Geometry check sheet. Reference: the model listing, model coordinates, mm. A direction names the side the tool comes from. Give positions to 0.01 mm unless a question says otherwise; leave off trailing zeros. Loops run counter-clockwise (first coordinate to the right, second up) from the corner with the lowest first, then second, coordinate; pieces in that order, holes last.
```python
from build123d import *

# Parameters (mm, degrees)
SKETCH1_R           = 11.1125
BOSS_EXTRUDE1_DEPTH = 18.415
SKETCH2_R           = 4.7625
BOSS_EXTRUDE2_DEPTH = 8.255
SKETCH3_R           = 3.175
BOSS_EXTRUDE3_DEPTH = 12.7
FILLET1_R           = 0.508
FILLET2_R           = 0.508


with BuildPart() as part:
    # Sketch1 → Boss-Extrude1 (new body)
    with BuildSketch(Plane(origin=(0, 0, 0), x_dir=(1, 0, 0), z_dir=(0, 1, 0))):
        with Locations(Location((0, 0, 0), (0, 0, 270))):
            Circle(SKETCH1_R)
    extrude(amount=BOSS_EXTRUDE1_DEPTH)

    # Sketch2 → Boss-Extrude2 (add)
    with BuildSketch(Plane(origin=(0, 18.415, 0), x_dir=(1, 0, 0), z_dir=(0, 1, 0))):
        with Locations(Location((0, 0, 0), (0, 0, 270))):
            Circle(SKETCH2_R)
    extrude(amount=BOSS_EXTRUDE2_DEPTH)

    # Sketch3 → Boss-Extrude3 (add)
    with BuildSketch(Plane(origin=(0, 26.67, 0), x_dir=(1, 0, 0), z_dir=(0, 1, 0))):
        with Locations(Location((0, 0, 0), (0, 0, 270))):
            Circle(SKETCH3_R)
    extrude(amount=BOSS_EXTRUDE3_DEPTH)

    # Fillet1
    fillet1_edges = [part.edges().sort_by_distance(p)[0] for p in [
        (0, 0, -11.1125),
        (0, 18.415, -11.1125),
    ]]
    fillet(fillet1_edges, radius=FILLET1_R)

    # Fillet2
    fillet2_edges = [part.edges().sort_by_distance(p)[0] for p in [
        (0, 39.37, -3.175),
    ]]
    fillet(fillet2_edges, radius=FILLET2_R)


solid = part.part
```
1) Sectioned sample at C-C on y = 5. Enter the section's corners in (x, z) (1 decimal).
2) Sectioned sample at D-D on y = 35. Enter the section's corners in (x, z) (3 decimals), plus the area to 3 significant figures.
3) Sectioned sample at A-A on x = 0. Enter the section's corners in (y, z) (1 decimal).
4) Depth check by flat-ended pin: P1, Ø6, axis at y = 34.5, z = 2.5, coming from the -X side (3 decimals); P2, Ø12, axis at x = -6.5, y = 12, coming from the +Z side; P3, Ø2, axis at x = 3, y = 4.5, coming from the -Z side; P4, Ø1, axis at x = -4, y = 31.5, coming from the -Z side. Enter the tip coordinate at first touch or a pass-through.
5) Scan lines: line 1 along Y through (x, z) = (-4.75, -9) (3 decimals); line 2 along X through (y, z) = (3.5, 8.5). Record each from-to range of solid material in increasing order.
6) Sectioned sample at B-B on z = 0. Enter the section's corners in (x, y) (1 decimal).
7) Tool access check on faces 1 (the cylindrical face through (-1.93, 32.68, -2.52)), 2 (the cylindrical face through (9.37, 9.086, 5.974)). Record the directions out of +Z, -Z, +X, -X, +Y, -Y that give a thin tool (end or side, any length) a straight path to the whole face; none if there is none.
Determined:
1. outline: circle Ø22.2 at (0, 0)
2. outline: circle Ø6.35 at (0, 0)
2. area: 31.7 mm2
3. outline: (0, -10.6) arc R0.5 ccw to (0.5, -11.1) - (17.9, -11.1) arc R0.5 ccw to (18.4, -10.6) - (18.4, -4.8) - (26.7, -4.8) - (26.7, -3.2) - (38.9, -3.2) arc R0.5 ccw to (39.4, -2.7) - (39.4, 2.7) arc R0.5 ccw to (38.9, 3.2) - (26.7, 3.2) - (26.7, 4.8) - (18.4, 4.8) - (18.4, 10.6) arc R0.5 ccw to (17.9, 11.1) - (0.5, 11.1) arc R0.5 ccw to (0, 10.6) - close
4. P1: stops at x = -3.175
4. P2: stops at z = 11.1
4. P3: stops at z = -10.93
4. P4: passes through
5. line 1: y = 0 to 18.415
5. line 2: x = -7.16 to 7.16
6. outline: (-11.1, 0.5) arc R0.5 ccw to (-10.6, 0) - (10.6, 0) arc R0.5 ccw to (11.1, 0.5) - (11.1, 17.9) arc R0.5 ccw to (10.6, 18.4) - (4.8, 18.4) - (4.8, 26.7) - (3.2, 26.7) - (3.2, 38.9) arc R0.5 ccw to (2.7, 39.4) - (-2.7, 39.4) arc R0.5 ccw to (-3.2, 38.9) - (-3.2, 26.7) - (-4.8, 26.7) - (-4.8, 18.4) - (-10.6, 18.4) arc R0.5 ccw to (-11.1, 17.9) - close
7. face 1: +Y
7. face 2: +Y, -Y
